Autodesk Inventor part; units mm, degrees
ref_plane "YZ Plane" through (0, 0, 0) normal (1, 0, 0) x (0, 1, 0)
ref_plane "XZ Plane" through (0, 0, 0) normal (0, 1, 0) x (-1, 0, 0)
ref_plane "XY Plane" through (0, 0, 0) normal (0, 0, 1) x (1, 0, 0)
sketch "スケッチ1" plane through (0, 0, 0) normal (1, 0, 0) x (0, 1, 0)
  line L0 (0, 0) -> (15, 0)
  line L1 (15, 0) -> (15, -10)
  line L2 (15, -10) -> (0, -10)
  line L3 (0, -10) -> (0, 0)
  line L4 (1, -1) -> (14, -1)
  line L5 (14, -1) -> (14, -9)
  line L6 (14, -9) -> (1, -9)
  line L7 (1, -9) -> (1, -1)
  dimension "d0" = 15
  dimension "d1" = 10
  dimension "d2" = 13
  dimension "d3" = 8
  dimension "d4" = 1
  dimension "d5" = 1
extrude "押し出し1" add sketch "スケッチ1" along normal blind 120
sketch "スケッチ2" plane through (0, 15, 0) normal (0, 1, 0) x (1, 0, 0)
  line L0 (0, 9) -> (0, 1)
  line L1 (0, 5) -> (120, 5)
  line L2 (120, 10) -> (120, 0)
  point P0 (0, 0)
  point P1 (5, 5)
  point P2 (115, 5)
  dimension "d8" = 5
  dimension "d9" = 5
hole "穴1" at (5, 15, -5) at (115, 15, -5) direction (0, -1, 0) diameter 3.2 end through all
properties part number "base_pipe1" material "アルミニウム 6061"
Model file for the job. Use its own axes, mm. A direction names the side the tool comes from. Give positions to 0.01 mm unless a question says otherwise; leave off trailing zeros. Loops run counter-clockwise (first coordinate to the right, second up) from the corner with the lowest first, then second, coordinate; pieces in that order, holes last. Notation, with made-up numbers: (13, -14) -> (72, -14) arc R11 ccw to (72, -10) -> close; hole circle Ø3 at (-10.75, 84). An arc over 180 degrees is marked (long way). Use a Markdown table: item, result. Add a question column.
(1) Tool access for faces 1 (the flat face through (59, 7, -1)), 2 (the cylindrical face through (4.93, 14.49, -6.6)): list every direction of +Z, -Z, +X, -X, +Y, -Y with a clear straight run to the whole face (end or side of a thin tool).
(2) Slice it at A-A on z = -8. List the corners of the cut face in (x, y), and give its area (3 significant figures).
(3) Mould opens along X. For faces 3 (the flat face through (59, 14, -5)), 4 (the cylindrical face through (113.414, 14.493, -5.208)), 5 (the flat face through (0, 7.4, -9.4)) say: +X half, -X half, draft (parallel to the pull), parting line (faces both ways), or undercut.
(4) Slice it at D-D on x = 5. List the corners of the cut face in (y, z).
(5) Drop flat-ended pins along their axis: pin 1 Ø3 at (x, z) = (5, -5) entering from +Y; pin 2 Ø5 at (x, z) = (79.5, -2) entering from -Y. Give the stop position or say it passes through.
(6) Slice it at C-C on y = 5.5. List the corners of the cut face in (x, z).
(7) Wall check: line 1 along X through (y, z) = (0.6, -5); line 2 along Y through (x, z) = (51, -8.75); line 3 along Z through (x, y) = (33, 5.5). Give the ranges that are in metal, low to high.
(8) Slice it at B-B on x = 19. List the corners of the cut face in (y, z).
Filled sheet:
| question | item | result |
|---|---|---|
| 1 | face 1 | +X, -X |
| 1 | face 2 | +Y, -Y |
| 2 | outline | (0, 0) -> (120, 0) -> (120, 1) -> (0, 1) -> close; (0, 14) -> (120, 14) -> (120, 15) -> (0, 15) -> close |
| 2 | area | 240 mm2 |
| 3 | face 3 | draft |
| 3 | face 4 | undercut |
| 3 | face 5 | -X half |
| 4 | outline | (0, -10) -> (15, -10) -> (15, -6.6) -> (14, -6.6) -> (14, -9) -> (1, -9) -> (1, -6.6) -> (0, -6.6) -> close; (0, -3.4) -> (1, -3.4) -> (1, -1) -> (14, -1) -> (14, -3.4) -> (15, -3.4) -> (15, 0) -> (0, 0) -> close |
| 5 | pin 1 | through |
| 5 | pin 2 | y = 0 |
| 6 | outline | (0, -10) -> (120, -10) -> (120, -9) -> (0, -9) -> close; (0, -1) -> (120, -1) -> (120, 0) -> (0, 0) -> close |
| 7 | line 1 | 0 to 3.4, 6.6 to 113.4, 116.6 to 120 |
| 7 | line 2 | 0 to 1, 14 to 15 |
| 7 | line 3 | -10 to -9, -1 to 0 |
| 8 | outline | (0, -10) -> (15, -10) -> (15, 0) -> (0, 0) -> close; hole (1, -9) -> (14, -9) -> (14, -1) -> (1, -1) -> close |
